Geometry check sheet. Reference: the model listing, model coordinates, mm. Face numbers are marked on the shaded views. A direction names the side the tool comes from. Give positions to 0.01 mm unless a question says otherwise; leave off trailing zeros. Order: outer loops, then holes, each group sorted by start corner. A loop starts at its lowest first (then second) coordinate and runs counter-clockwise, first axis right, second up. Notation, with made-up numbers: M 80,60.25 L 91,60.25 A13 ccw 91,79.25 Z; hole C 48,-18 d11. An arc over 180 degrees is marked long. Answer as CSV lines item,"result".
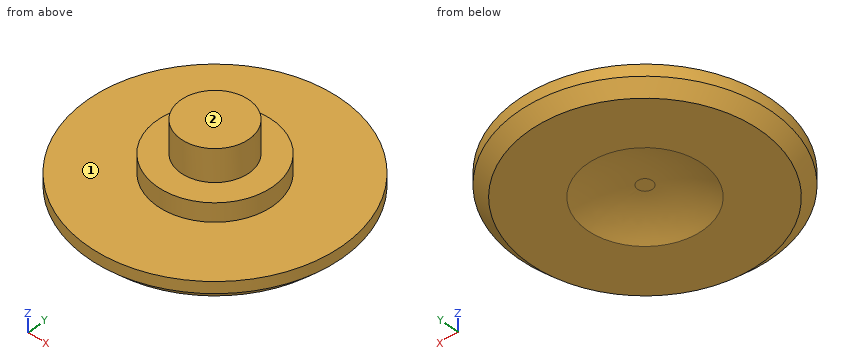
from build123d import *

# Parameters (mm, degrees)
F0_R     = 11
F0_R_2   = 5
F1_DEPTH = 2
F0_R_3   = 2.95
F2_DEPTH = 3.6
F0_R_4   = 1.8
F3_DEPTH = 6.4
F4_DEPTH = 1
F5_SIZE  = 1


# Not quite as in the source:
# - a fillet or chamfer that OpenCascade refuses, or shapes differently, is made with other operations: its cross-section is extruded or revolved along the edge and cut away or added
# - a feature of the source that left no trace in its solid (it failed there, or was rolled back) is left out


with BuildPart() as f1:
    # F0 (on Top) → F1 (new body)
    with BuildSketch(Plane.XY):
        Circle(F0_R)
        Circle(F0_R_2, mode=Mode.SUBTRACT)
    extrude(amount=F1_DEPTH)

    # F0 (on Top) → F2 (join)
    with BuildSketch(Plane.XY):
        Circle(F0_R_2)
        Circle(F0_R_3, mode=Mode.SUBTRACT)
    extrude(amount=F2_DEPTH)

    # F0 (on Top) → F3 (join)
    with BuildSketch(Plane.XY):
        Circle(F0_R_3)
        Circle(F0_R_4, mode=Mode.SUBTRACT)
        Circle(F0_R_4)
    extrude(amount=F3_DEPTH)

    # F0 (on Top) → F4 (cut)
    with BuildSketch(Plane.XY):
        Circle(F0_R_2)
        Circle(F0_R_3, mode=Mode.SUBTRACT)
        Circle(F0_R_3)
        Circle(F0_R_4, mode=Mode.SUBTRACT)
        Circle(F0_R_4)
    extrude(amount=F4_DEPTH, mode=Mode.SUBTRACT)

    # F5
    f5_edges = [f1.edges().sort_by_distance(p)[0] for p in [
        (-11, 0, 0),
    ]]
    chamfer(f5_edges, length=F5_SIZE)

    # F6: fillet of radius 10 on 1 edges, made by hand

    # F6_s1 → F6_t2 (revolve)
    with BuildSketch(Plane.XZ):
        with BuildLine():
            ThreePointArc((5, 0), (2.877169034, 0.7467943448), (0.6411010565, 1))
            Line((0.6411010565, 1), (5, 1))
            Line((5, 1), (5, 0))
        make_face()
    revolve(axis=Axis((0, 0, 1), (0, 0, 1)))


solid = f1.part
(1) Material ranges on line 1 (Z direction, x = -3.5, y = -7.25); line 2 (Z direction, x = -9.25, y = -5.25); line 3 (X direction, y = 5.5, z = 1.25), recorded low to high.
The answers:
line 1,"z = 0 to 2"
line 2,"z = 0.64 to 2"
line 3,"x = -9.53 to 9.53"
(2) Gauge pin test, flat ends, axial feed: P1, Ø11, axis at x = 5.5, y = -4.5, coming from the +Z side; P2, Ø1.4, axis at x = 0, y = 0, coming from the -Z side; P3, Ø1.5, axis at x = -1.5, z = 4, coming from the -Y side. Record the tip position at first contact, or that the pin passes through.
The answers:
P1,"stops at z = 6.4"
P2,"stops at z = 1"
P3,"stops at y = -4.92"
(3) Tool access check on the marked faces 1 and 2. Record the directions out of +Z, -Z, +X, -X, +Y, -Y that give a thin tool (end or side, any length) a straight path to the whole face; none if there is none.
The answers:
face 1,"+Z"
face 2,"+Z, +X, -X, +Y, -Y"
(4) Section check A-A on z = 3.25. Enter the section's corners in (x, y), then the cut area to 3 significant figures.
The answers:
outline,"C 0,0 d10"
area,"78.5 mm2"
